Read the model definition and answer for the solid it produces. Units are mm, in the model's axes. A direction names the side the tool comes from. Round coordinates to 2 decimals unless told otherwise and drop trailing zeros. Order: outer loops, then holes, each group sorted by start corner. A loop starts at its lowest first (then second) coordinate and runs counter-clockwise, first axis right, second up. Notation, with made-up numbers: (-29, 22) -> (-2, 22) arc R24 ccw to (-2, 57) -> close; hole circle Ø3 at (-6.75, 35.25). An arc over 180 degrees is marked (long way). Answer as a JSON object with one key per item and string values. Group by question number.
Item 1: Section C-C, the plane y = 3.5 is taken. Write down the section's boundary in (x, z), plus the area to 3 significant figures.
Item 2: The mould has two halves that part along X. Classify faces 1 (the flat face through (0.02, 5, -0.31)), 2 (the flat face through (-3.77, 6.97, 2.13)), 3 (the flat face through (1, 5, -3)), 4 (the cylindrical face through (0.45, 2.46, -1.43)): pulls with the +X half, pulls with the -X half, needs draft (parallel to the pull), parting line crosses it, or undercut.
Item 3: Consider probe 1 along X at (y, z) = (2.75, 0); probe 2 along X at (y, z) = (4.5, 1.25); probe 3 along Y at (x, z) = (-0.5, 4). Determine where each line is inside the solid, lowest interval first. Write a range as from..to.
Item 4: Section A-A, the plane y = 8.75 is taken. Write down the section's boundary in (x, z).
Item 5: For faces 5 (the cylindrical face through (0.9, 2.46, 2.86)), 6 (the flat face through (4.1, 9, -0.7)), 7 (the flat face through (3.77, 6.97, -2.13)), determine the directions among +Z, -Z, +X, -X, +Y, -Y from which every point of the face is accessible in a straight line to the end or side of a thin tool.
Item 6: Section B-B, the plane x = 0 is taken. Write down the section's boundary in (y, z).
Item 7: Given P1, Ø2.5, axis at x = 0, z = 0, coming from the -Y side; P2, Ø4.5, axis at x = 2, z = -1, coming from the +Y side; P3, Ø1.5, axis at x = 2.5, z = 0, coming from the +Y side, each flat-ended and moving along its own axis, determine where each tip first touches the part or whether it passes through.
from build123d import *

# Parameters (mm, degrees)
SKETCH1_R           = 3
BOSS_EXTRUDE1_DEPTH = 5
BOSS_EXTRUDE2_DEPTH = 4
SKETCH4_R           = 1
BOSS_EXTRUDE4_DEPTH = 3
DRAFT4_ANGLE        = 45
SKETCH5_R           = 0.15
CUT_EXTRUDE1_DEPTH  = 50
SKETCH6_R           = 1.5
CUT_EXTRUDE2_DEPTH  = 5


with BuildPart() as part:
    # Sketch1 → Boss-Extrude1 (new body)
    with BuildSketch(Plane(origin=(0, 0, 0), x_dir=(1, 0, 0), z_dir=(0, 1, 0))):
        with Locations(Location((0, 0, 0), (0, 0, 270))):
            Circle(SKETCH1_R)
    extrude(amount=BOSS_EXTRUDE1_DEPTH)

    # Sketch2 → Boss-Extrude2 (add)
    with BuildSketch(Plane(origin=(0, 5, 0), x_dir=(1, 0, 0), z_dir=(0, 1, 0))):
        Polygon((5, 0), (2.5, 4.330127019), (-2.5, 4.330127019), (-5, 0), (-2.5, -4.330127019), (2.5, -4.330127019), align=None)
    extrude(amount=BOSS_EXTRUDE2_DEPTH)

    # Sketch4 → Boss-Extrude4 (add)
    with BuildSketch(Plane(origin=(0, 9, 0), x_dir=(1, 0, 0), z_dir=(0, 1, 0))):
        with Locations(Location((0, 0, 0), (0, 0, 270))):
            Circle(SKETCH4_R)
    extrude(amount=BOSS_EXTRUDE4_DEPTH)

    # Draft4
    draft4_faces = [part.faces().sort_by_distance(p)[0] for p in [
        (0, 10.5, -1),
    ]]
    draft(draft4_faces, Plane.ZX.offset(12), DRAFT4_ANGLE)

    # Sketch5 → Cut-Extrude1 (cut)
    with BuildSketch(Plane(origin=(0, 12, 0), x_dir=(1, 0, 0), z_dir=(0, 1, 0))):
        with Locations(Location((0, 0, 0), (0, 0, 270))):
            Circle(SKETCH5_R)
    extrude(amount=-CUT_EXTRUDE1_DEPTH, mode=Mode.SUBTRACT)

    # Sketch6 → Cut-Extrude2 (cut)
    with BuildSketch(Plane.XZ):
        with Locations(Location((0, 0, 0), (0, 0, 270))):
            Circle(SKETCH6_R)
    extrude(amount=-CUT_EXTRUDE2_DEPTH, mode=Mode.SUBTRACT)


solid = part.part
Values found:
{
 "1": {"outline": "circle Ø6 at (0, 0); hole circle Ø3 at (0, 0)", "area": "21.2 mm2"},
 "2": {"face 1": "undercut", "face 2": "pulls with the -X half", "face 3": "needs draft", "face 4": "undercut"},
 "3": {"probe 1": "-3..-1.5, 1.5..3", "probe 2": "-2.73..-0.83, 0.83..2.73", "probe 3": "5..9"},
 "4": {"outline": "(-5, 0) -> (-2.5, -4.33) -> (2.5, -4.33) -> (5, 0) -> (2.5, 4.33) -> (-2.5, 4.33) -> close; hole circle Ø0.3 at (0, 0)"},
 "5": {"face 5": "-Y", "face 6": "+Y", "face 7": "-Z, +X, +Y, -Y"},
 "6": {"outline": "(0, -3) -> (5, -3) -> (5, -4.33) -> (9, -4.33) -> (9, -4) -> (12, -1) -> (12, -0.15) -> (5, -0.15) -> (5, -1.5) -> (0, -1.5) -> close; (0, 1.5) -> (5, 1.5) -> (5, 0.15) -> (12, 0.15) -> (12, 1) -> (9, 4) -> (9, 4.33) -> (5, 4.33) -> (5, 3) -> (0, 3) -> close"},
 "7": {"P1": "y = 5", "P2": "y = 12", "P3": "y = 11.25"}
}
